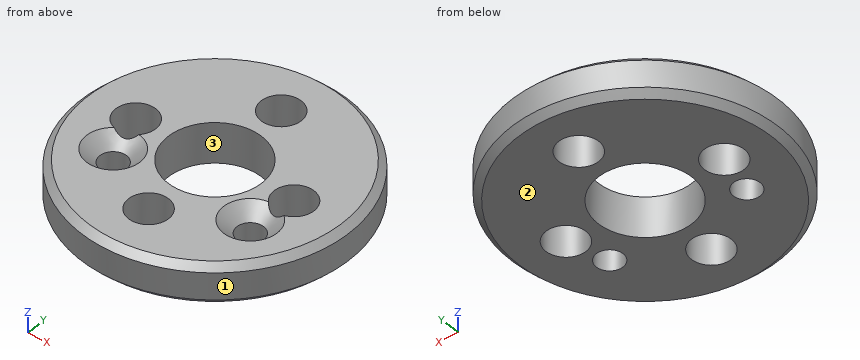
from build123d import *

# Parameters (mm, degrees)
SKETCH_1_R      = 10
SKETCH_1_R_2    = 1.5
SKETCH_1_R_3    = 3.5
SKETCH_1_R_4    = 1
EXTRUDE_1_DEPTH = 3
CHAMFER_1_SIZE  = 0.5
CHAMFER_2_SIZE  = 1


with BuildPart() as part:
    # 草图1 → 凸台-拉伸1 (new body)
    with BuildSketch(Plane.XY):
        Circle(SKETCH_1_R)
        with Locations((-6, 0)):
            Circle(SKETCH_1_R_2, mode=Mode.SUBTRACT)
        with Locations((0, -6)):
            Circle(SKETCH_1_R_2, mode=Mode.SUBTRACT)
        with Locations((6, 0)):
            Circle(SKETCH_1_R_2, mode=Mode.SUBTRACT)
        Circle(SKETCH_1_R_3, mode=Mode.SUBTRACT)
        with Locations((0, 6)):
            Circle(SKETCH_1_R_2, mode=Mode.SUBTRACT)
        with Locations((5.196152423, -3)):
            Circle(SKETCH_1_R_4, mode=Mode.SUBTRACT)
        with Locations((-5.196152423, -3)):
            Circle(SKETCH_1_R_4, mode=Mode.SUBTRACT)
    extrude(amount=EXTRUDE_1_DEPTH)

    # 倒角1
    chamfer_1_edges = [part.edges().sort_by_distance(p)[0] for p in [
        (-10, 0, 0),
        (-10, 0, 3),
    ]]
    chamfer(chamfer_1_edges, length=CHAMFER_1_SIZE)

    # 倒角2
    # the kernel refuses this chamfer: 1 mm, written as the material it takes off along each edge
    with BuildSketch(Plane(origin=(5.196152423, -3, 3), x_dir=(1, 0, 0), z_dir=(0, -1, 0))) as chamfer_2_piece_1:
        Polygon((1 + CHAMFER_2_SIZE, 0), (1, -CHAMFER_2_SIZE), (1, 0), align=None)
    revolve(axis=Axis((5.196152423, -3, 3), (0, 0, 1)), mode=Mode.SUBTRACT)
    with BuildSketch(Plane(origin=(-5.196152423, -3, 3), x_dir=(1, 0, 0), z_dir=(0, -1, 0))) as chamfer_2_piece_2:
        Polygon((1 + CHAMFER_2_SIZE, 0), (1, -CHAMFER_2_SIZE), (1, 0), align=None)
    revolve(axis=Axis((-5.196152423, -3, 3), (0, 0, 1)), mode=Mode.SUBTRACT)


solid = part.part
Design review of the part built by this model. Coordinates are the model's own, in mm. Face numbers are marked on the shaded views. Coordinates: 2 decimals unless noted, no trailing zeros. Loops run counter-clockwise (first coordinate to the right, second up) from the corner with the lowest first, then second, coordinate; pieces in that order, holes last. Notation, with made-up numbers: (42, 2) -> (55, 2) arc R17 cw to (55, 16) -> close; hole circle Ø6 at (25, 82.25). An arc over 180 degrees is marked (long way). Use a Markdown table: item, result. Add a question column.
Item 1: The part is to be moulded in two halves that separate along X. For the marked faces 1, 2 and 3, say which applies: +X half, -X half, draft (parallel to the pull), parting line (faces both ways), or undercut.
Item 2: Clearance check with flat-ended pins moving along their axes: P1, Ø1, axis at x = -5.5, z = 2, coming from the -Y side; P2, Ø1.2, axis at x = 5.2, y = -3, coming from the +Z side. State where each tip first meets the part, or that it passes through.
Item 3: We need section A-A, the plane x = 0. Write out the cut boundary in (y, z), and give its area (3 significant figures).
Item 4: We need section B-B, the plane z = 1.15. Write out the cut boundary in (x, y).
Item 5: We need section C-C, the plane y = -3. Count the separate pieces of the cut face and the enclosed holes in it, and give its area (3 significant figures).
Item 6: Wall thickness on L1, parallel to Y at x = 0, z = 1.45; L2, parallel to X at y = -2.5, z = 1.8; L3, parallel to Y at x = 6, z = 1.8: over which ranges is each line inside the solid? List them lowest first. Write a range as from..to.
Numbers:
| question | item | result |
|---|---|---|
| 1 | face 1 | parting line |
| 1 | face 2 | draft |
| 1 | face 3 | undercut |
| 2 | P1 | stops at y = -8.66 |
| 2 | P2 | passes through |
| 3 | outline | (-10, 0.5) -> (-9.5, 0) -> (-7.5, 0) -> (-7.5, 3) -> (-9.5, 3) -> (-10, 2.5) -> close; (-4.5, 0) -> (-3.5, 0) -> (-3.5, 3) -> (-4.5, 3) -> close; (3.5, 0) -> (4.5, 0) -> (4.5, 3) -> (3.5, 3) -> close; (7.5, 0) -> (9.5, 0) -> (10, 0.5) -> (10, 2.5) -> (9.5, 3) -> (7.5, 3) -> close |
| 3 | area | 20.5 mm^2 |
| 4 | outline | circle Ø20 at (0, 0); hole circle Ø3 at (-6, 0); hole circle Ø2 at (-5.2, -3); hole circle Ø7 at (0, 0); hole circle Ø3 at (0, -6); hole circle Ø3 at (0, 6); hole circle Ø2 at (5.2, -3); hole circle Ø3 at (6, 0) |
| 5 | separate pieces | 4 |
| 5 | enclosed holes | 0 |
| 5 | area | 31.9 mm^2 |
| 6 | L1 | y = -10..-7.5, -4.5..-3.5, 3.5..4.5, 7.5..10 |
| 6 | L2 | x = -9.68..-6.06, -4.33..-2.45, 2.45..4.33, 6.06..9.68 |
| 6 | L3 | y = -8..-3.59, -2.41..-1.5, 1.5..8 |
